The model under review builds one solid part; all positions refer to its coordinate system, in mm. A direction names the side the tool comes from. Round coordinates to 2 decimals unless told otherwise and drop trailing zeros. Write each loop counter-clockwise with the first axis right and the second up, starting at its lowest first coordinate (ties: lowest second). Pieces come first, ordered by that corner, then holes. Notation, with made-up numbers: M 81,-29.75 L 127,-29.75 A14 cw 127,-22.75 Z; hole C 60,-36.75 d8. An arc over 180 degrees is marked long. One line per item, written item: value. Start each with the question number.
1) Mouldability with a two-part tool opening along X and no side actions: class faces 5 (the face through (0, -69, -29)), 6 (the face through (3, -59.83, -29)), 7 (the face through (-6, -70, 19)), 8 (the face through (10, 46, 9)) as +X half, -X half, draft (parallel to the pull), parting line (faces both ways), or undercut.
2) Tool access review of faces 1 (the face through (6, -70, 19)), 2 (the face through (6, -66, -26)), 3 (the face through (11, -74.83, 30)), 4 (the face through (0, -74.83, -20)): name each direction out of +Z, -Z, +X, -X, +Y, -Y from which nothing blocks a thin tool from reaching the whole face with its end or side.
3) For P1, Ø1.6, axis at y = -67.5, z = 19, coming from the +X side; P2, Ø1.5, axis at x = 10, y = 20, coming from the -Z side; P3, Ø10, axis at x = -5.5, y = 18, coming from the +Z side; P4, Ø6, axis at y = 38, z = 8.5, coming from the +X side, all flat-tipped, find the tip position at first contact; note any pin that passes through.
4) Wall thickness on probe 1 along X at (y, z) = (-69.5, -25.5); probe 2 along X at (y, z) = (-27, 5.5); probe 3 along X at (y, z) = (18.5, 3): over which ranges is each line inside the solid? List them lowest first.
5) Take a section at C-C, the plane x = 12.5. Write out the cut boundary in (y, z), and give its area (3 significant figures).
6) Take a section at A-A, the plane z = 0. Write out the cut boundary in (x, y), and give its area (3 significant figures).
7) Take a section at D-D, the plane y = 44.5. Write out the cut boundary in (x, z), and give its area (3 significant figures).
8) Take a section at B-B, the plane y = -66. Write out the cut boundary in (x, z), and give its area (3 significant figures).
from build123d import *

# Parameters (mm, degrees)
SKETCH3_R           = 12.5
SKETCH3_R_2         = 9
BOSS_EXTRUDE2_DEPTH = 10
BOSS_EXTRUDE3_DEPTH = 15
BOSS_EXTRUDE4_DEPTH = 7.5
SKETCH4_W           = 6
SKETCH4_H           = 8.322914524
BOSS_EXTRUDE5_DEPTH = 15
SKETCH5_R           = 3.25
CUT_EXTRUDE1_DEPTH  = 122.045487318
CUT_EXTRUDE3_DEPTH  = 5


with BuildPart() as part:
    # Sketch3 → Boss-Extrude2 (new, symmetric)
    with BuildSketch(Plane(origin=(0, 0, 0), x_dir=(0, 0, -1), z_dir=(1, 0, 0))):
        with Locations((0, 42.570273578)):
            Circle(SKETCH3_R)
        with Locations((0, 42.570273578)):
            Circle(SKETCH3_R_2, mode=Mode.SUBTRACT)
    extrude(amount=BOSS_EXTRUDE2_DEPTH, both=True)



with BuildPart() as body_2:
    # Sketch3_4 → Boss-Extrude3 (new, symmetric)
    with BuildSketch(Plane(origin=(0, 0, 0), x_dir=(0, 0, -1), z_dir=(1, 0, 0))):
        with BuildLine():
            Line((0, -55.329726422), (0, -52.329726422))
            ThreePointArc((0, -52.329726422), (-6.05446696, -53.058908312), (-11.762674496, -55.204751534))
            ThreePointArc((-11.762674496, -55.204751534), (-20.979040447, -63.333869707), (-25.322914524, -74.829726422))
            Line((-25.322914524, -74.829726422), (-35, -74.829726422))
            Line((-35, -74.829726422), (-35, -77.829726422))
            Line((-35, -77.829726422), (-22.5, -77.829726422))
            ThreePointArc((-22.5, -77.829726422), (-15.909902577, -61.919823845), (0, -55.329726422))
        make_face()
        with BuildLine():
            ThreePointArc((11.762674496, -55.204751534), (6.05446696, -53.058908312), (0, -52.329726422))
            Line((0, -52.329726422), (0, -55.329726422))
            ThreePointArc((0, -55.329726422), (15.909902577, -61.919823845), (22.5, -77.829726422))
            Line((22.5, -77.829726422), (35, -77.829726422))
            Line((35, -77.829726422), (35, -74.829726422))
            Line((35, -74.829726422), (25.322914524, -74.829726422))
            ThreePointArc((25.322914524, -74.829726422), (20.979040447, -63.333869707), (11.762674496, -55.204751534))
        make_face()
    extrude(amount=BOSS_EXTRUDE3_DEPTH, both=True)


with BuildPart() as part_1:
    add(part.part)

    add(body_2.part)  # Boss-Extrude4 merges body 2
    # Sketch3_5 → Boss-Extrude4 (add, symmetric)
    with BuildSketch(Plane(origin=(0, 0, 0), x_dir=(0, 0, -1), z_dir=(1, 0, 0))):
        with BuildLine():
            Line((0, -52.329726422), (0, 30.070273578))
            ThreePointArc((0, 30.070273578), (-2.15073746, 30.256690493), (-4.237325504, 30.810381037))
            Line((-4.237325504, 30.810381037), (-11.762674496, -55.204751534))
            ThreePointArc((-11.762674496, -55.204751534), (-6.05446696, -53.058908312), (0, -52.329726422))
        make_face()
        with BuildLine():
            ThreePointArc((4.237325504, 30.810381037), (2.15073746, 30.256690493), (0, 30.070273578))
            Line((0, 30.070273578), (0, -52.329726422))
            ThreePointArc((0, -52.329726422), (6.05446696, -53.058908312), (11.762674496, -55.204751534))
            Line((11.762674496, -55.204751534), (4.237325504, 30.810381037))
        make_face()
    extrude(amount=BOSS_EXTRUDE4_DEPTH, both=True)

    # Sketch4 → Boss-Extrude5 (add)
    with BuildSketch(Plane(origin=(0, -74.829726422, 0), x_dir=(1, 0, 0), z_dir=(0, 1, 0))):
        with BuildLine():
            Line((0, 25.322914524), (0, 35))
            ThreePointArc((0, 35), (-4.242640687, 33.242640687), (-6, 29))
            Line((-6, 29), (-6, 25.322914524))
            Line((-6, 25.322914524), (0, 25.322914524))
        make_face()
        with BuildLine():
            ThreePointArc((6, 29), (4.242640687, 33.242640687), (0, 35))
            Line((0, 35), (0, 25.322914524))
            Line((0, 25.322914524), (6, 25.322914524))
            Line((6, 25.322914524), (6, 29))
        make_face()
        with Locations((3, 21.161457262)):
            Rectangle(SKETCH4_W, SKETCH4_H)
        with Locations((-3, 21.161457262)):
            Rectangle(SKETCH4_W, SKETCH4_H)
    boss_extrude5 = extrude(amount=BOSS_EXTRUDE5_DEPTH)

    # Sketch5 → Cut-Extrude1 (cut, through all)
    with BuildSketch(Plane(origin=(0, -59.829726422, 0), x_dir=(1, 0, 0), z_dir=(0, 1, 0))):
        with Locations(Location((0, 25.75, 0), (0, 0, 270))):
            Circle(SKETCH5_R)
    cut_extrude1 = extrude(amount=-CUT_EXTRUDE1_DEPTH, mode=Mode.SUBTRACT)

    # Mirror1: Boss-Extrude5, Cut-Extrude1 across plane
    add(boss_extrude5.mirror(Plane.XY))
    add(cut_extrude1.mirror(Plane.XY), mode=Mode.SUBTRACT)

    # Sketch9 → Cut-Extrude3 (cut)
    with BuildSketch(Plane.ZY.offset(7.5)):
        with BuildLine():
            ThreePointArc((-1.546317924, 27.147598684), (0, 27.070273578), (1.546317924, 27.147598684))
            Line((1.546317924, 27.147598684), (8.346541197, -50.579308993))
            ThreePointArc((8.346541197, -50.579308993), (0, -49.329726422), (-8.346541197, -50.579308993))
            Line((-8.346541197, -50.579308993), (-1.546317924, 27.147598684))
        make_face()
    cut_extrude3 = extrude(amount=-CUT_EXTRUDE3_DEPTH, mode=Mode.SUBTRACT)

    # Mirror2: Cut-Extrude3 across plane
    add(cut_extrude3.mirror(Plane(origin=(0, 0, 0), x_dir=(0, 0, 1), z_dir=(1, 0, 0))), mode=Mode.SUBTRACT)


solid = part_1.part
Checked values:
1. face 5: undercut
1. face 6: draft
1. face 7: -X half
1. face 8: +X half
2. face 1: +X, -Y
2. face 2: -Z, +X, +Y
2. face 3: +Z, +X, +Y
2. face 4: +X, -X, -Y
3. P1: stops at x = 6
3. P2: passes through
3. P3: stops at z = 5.8
3. P4: stops at x = 10
4. probe 1: x = -6 to -3.24, 3.24 to 6
4. probe 2: x = -2.5 to 2.5
4. probe 3: x = -7.5 to 7.5
5. outline: M -77.83,-35 L -74.83,-35 L -74.83,-25.32 A25.5 ccw -74.83,25.32 L -74.83,35 L -77.83,35 L -77.83,22.5 A22.5 cw -77.83,-22.5 Z
5. area: 284 mm2
6. outline: M -15,-55.33 L 15,-55.33 L 15,-52.33 L 7.5,-52.33 L 7.5,-49.33 L 2.5,-49.33 L 2.5,27.07 L 7.5,27.07 L 7.5,30.07 L 10,30.07 L 10,33.57 L -10,33.57 L -10,30.07 L -7.5,30.07 L -7.5,27.07 L -2.5,27.07 L -2.5,-49.33 L -7.5,-49.33 L -7.5,-52.33 L -15,-52.33 Z; M -10,51.57 L 10,51.57 L 10,55.07 L -10,55.07 Z
6. area: 702 mm2
7. outline: M -10,-12.35 L 10,-12.35 L 10,-8.79 L -10,-8.79 Z; M -10,8.79 L 10,8.79 L 10,12.35 L -10,12.35 Z
7. area: 142 mm2
8. outline: M -15,-22.59 L -6,-22.59 L -6,-29 A6 ccw 6,-29 L 6,-22.59 L 15,-22.59 L 15,-19.14 L 6,-19.14 L 6,-17 L -6,-17 L -6,-19.14 L -15,-19.14 Z; M -15,19.14 L -6,19.14 L -6,17 L 6,17 L 6,19.14 L 15,19.14 L 15,22.59 L 6,22.59 L 6,29 A6 ccw -6,29 L -6,22.59 L -15,22.59 Z; hole C 0,-25.75 d6.5; hole C 0,25.75 d6.5
8. area: 459 mm2
